```python
from build123d import *

# Parameters (mm, degrees)
CUT_EXTRUDE1_DEPTH      = 22.485343842
CUT_EXTRUDE1_DEPTH_BACK = 22.485343842
SKETCH4_R               = 1


with BuildPart() as part:
    # Sketch1 → Revolve1 (revolve)
    with BuildSketch(Plane.XY, mode=Mode.PRIVATE) as revolve1_sk:
        Polygon((0, 0), (8, 0), (8, 1.6), (4.8, 1.6), (4.8, 5.6), (0.8, 5.6), (0.8, 9.6), (0, 9.6), align=None)
    revolve(revolve1_sk.sketch.rotate(Axis((124.631559107, -4.5, 0), (-1, 0, 0)), 90), axis=Axis((124.631559107, -4.5, 0), (-1, 0, 0)))

    # Sketch4 → Cut-Extrude1 (cut, two sides: drawn at the far end of the back side and taken through both)
    with BuildSketch(Plane(origin=(0, -4.5, 0), x_dir=(1, 0, 0), z_dir=(0, 1, 0)).offset(-CUT_EXTRUDE1_DEPTH_BACK)):
        with Locations(Location((3.05, 0, 0), (0, 0, 270))):
            Circle(SKETCH4_R)
    extrude(amount=CUT_EXTRUDE1_DEPTH + CUT_EXTRUDE1_DEPTH_BACK, mode=Mode.SUBTRACT)


solid = part.part
```
The listing builds one solid part. Answer for the finished solid, in the listing's coordinates (mm). A direction names the side the tool comes from. Give positions to 0.01 mm unless a question says otherwise; leave off trailing zeros. Order: outer loops, then holes, each group sorted by start corner. A loop starts at its lowest first (then second) coordinate and runs counter-clockwise, first axis right, second up. Notation, with made-up numbers: (12, 73.25) - (19, 73.25) arc R27 cw to (19, 106.25) - close; hole circle Ø1 at (81.25, -26). An arc over 180 degrees is marked (long way). Use one line per item in the form item = value. Start each with the question number.
(1) Flat-ended cylindrical pins translate along their axes: pin 1 Ø4 at (x, y) = (3, 0) entering from -Z; pin 2 Ø2.5 at (x, z) = (3.05, 0) entering from +Y; pin 3 Ø2.5 at (x, z) = (3.05, 0) entering from -Y. Find the tip coordinate at first contact, or state that the pin passes through.
(2) The mould has two halves that part along X. Classify faces 1 (the flat face through (0.8, -8, -10)), 2 (the cylindrical face through (2.074, -11.782, -0.217)), 3 (the cylindrical face through (6.378, -9.644, -3.279)): released by +X, released by -X, zero draft, split by the parting line, or undercut.
(3) A cutting plane is placed at C-C, the plane x = 3.05. Write down the section's boundary in (y, z).
(4) For faces 4 (the flat face through (0, -7.8, 3.3)), 5 (the flat face through (4.8, 2, 0)), determine the directions among +Z, -Z, +X, -X, +Y, -Y from which every point of the face is accessible in a straight line to the end or side of a thin tool.
(5) Consider line 1 (Y direction, x = 5.75, z = 0); line 2 (X direction, y = -12.9, z = 0); line 3 (X direction, y = -4.25, z = -11). Determine where each line is inside the solid, lowest interval first. Write a range as from..to.
(6) A cutting plane is placed at B-B, the plane z = 0. Write down the section's boundary in (x, y), then the cut area to 3 significant figures.
(7) A cutting plane is placed at D-D, the plane z = -3.75. Write down the section's boundary in (x, y), then the cut area to 3 significant figures.
(8) A cutting plane is placed at A-A, the plane y = -4.5. Write down the section's boundary in (x, z), then the cut area to 3 significant figures.
Ans:
q1.pin_1 = -9.79
q1.pin_2 = 5.6
q1.pin_3 = -14.6
q2.face_1 = released by +X
q2.face_2 = undercut
q2.face_3 = zero draft
q3.outline = (-14.55, -1) arc R10.1 ccw to (5.55, -1) - (-0.11, -1) arc R4.5 cw to (-8.89, -1) - close; (-14.55, 1) - (-8.89, 1) arc R4.5 cw to (-0.11, 1) - (5.55, 1) arc R10.1 ccw to start
q4.face_4 = +Z, -Z, -X, +Y, -Y
q4.face_5 = +X
q5.line_1 = -10.6..-9, 0..1.6
q5.line_2 = 0..2.05, 4.05..4.8
q5.line_3 = 0..0.8
q6.outline = (0, -18.6) - (0.8, -18.6) - (0.8, -14.6) - (2.05, -14.6) - (2.05, -9) - (0, -9) - close; (0, 0) - (2.05, 0) - (2.05, 5.6) - (0.8, 5.6) - (0.8, 9.6) - (0, 9.6) - close; (4.05, -14.6) - (4.8, -14.6) - (4.8, -10.6) - (8, -10.6) - (8, -9) - (4.05, -9) - close; (4.05, 0) - (8, 0) - (8, 1.6) - (4.8, 1.6) - (4.8, 5.6) - (4.05, 5.6) - close
q6.area = 48.0 mm^2
q7.outline = (0, -18.09) - (0.8, -18.09) - (0.8, -13.88) - (4.8, -13.88) - (4.8, -9.31) - (8, -9.31) - (8, -6.99) - (0, -6.99) - close; (0, -2.01) - (8, -2.01) - (8, 0.31) - (4.8, 0.31) - (4.8, 4.88) - (0.8, 4.88) - (0.8, 9.09) - (0, 9.09) - close
q7.area = 87.8 mm^2
q8.outline = (0, -14.1) - (0.8, -14.1) - (0.8, -10.1) - (4.8, -10.1) - (4.8, -6.1) - (8, -6.1) - (8, -4.5) - (0, -4.5) - close; (0, 4.5) - (8, 4.5) - (8, 6.1) - (4.8, 6.1) - (4.8, 10.1) - (0.8, 10.1) - (0.8, 14.1) - (0, 14.1) - close
q8.area = 70.4 mm^2
